Could you check a few things on this model? Use its own coordinates, in mm. Face numbers are marked on the shaded views. A direction names the side the tool comes from. Round coordinates to 2 decimals unless told otherwise and drop trailing zeros. Loops run counter-clockwise (first coordinate to the right, second up) from the corner with the lowest first, then second, coordinate; pieces in that order, holes last. Notation, with made-up numbers: (37, 46.25) -> (46, 46.25) arc R26 ccw to (46, 74.25) -> close; hole circle Ø3 at (83, -14). An arc over 180 degrees is marked (long way). One line per item, written item: value.
from build123d import *

# Parameters (mm, degrees)
P_IDAT_VYSUNUT_M2_DEPTH = 8


with BuildPart() as part:
    # Skica1 → Přidat vysunutím2 (new body)
    with BuildSketch(Plane(origin=(0, 0, 0), x_dir=(1, 0, 0), z_dir=(0, 1, 0))):
        with BuildLine():
            Line((0, -10), (0, 10))
            Line((0, 10), (5, 15))
            Line((5, 15), (36, 15))
            ThreePointArc((36, 15), (38.828427125, 16.171572875), (40, 19))
            Line((40, 19), (40, 25))
            Line((40, 25), (30, 25))
            Line((30, 25), (30, 20))
            Line((30, 20), (-13.506811582, 29.645227916))
            ThreePointArc((-13.506811582, 29.645227916), (-38.916330448, 23.640944379), (-49.997883531, 0))
            ThreePointArc((-49.997883531, 0), (-38.916330448, -23.640944379), (-13.506811582, -29.645227916))
            Line((-13.506811582, -29.645227916), (30, -20))
            Line((30, -20), (30, -25))
            Line((30, -25), (40, -25))
            Line((40, -25), (40, -19))
            ThreePointArc((40, -19), (38.828427125, -16.171572875), (36, -15))
            Line((36, -15), (5, -15))
            Line((5, -15), (0, -10))
        make_face()
    extrude(amount=P_IDAT_VYSUNUT_M2_DEPTH)


solid = part.part
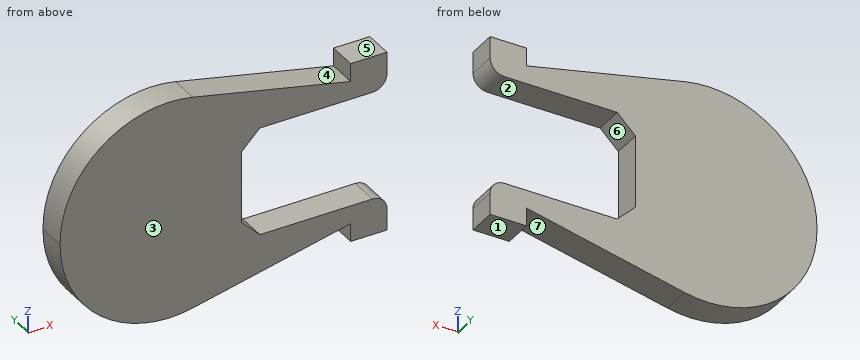
(1) If I drill on L1, parallel to Z at x = 31.5, y = 4.75; L2, parallel to X at y = 6, z = 0.5; L3, parallel to X at y = 4.75, z = 18, over which ranges is the centre line in solid material (lowest first)?
Recorded:
L1: -25 to -15, 15 to 25
L2: -50 to 0
L3: -44.26 to 39.87
(2) If we section it at A-A, the plane x = 34.5: Please give me the cut outline in (y, z).
Recorded:
outline: (0, -25) -> (8, -25) -> (8, -15) -> (0, -15) -> close; (0, 15) -> (8, 15) -> (8, 25) -> (0, 25) -> close
(3) If we section it at C-C, the plane y = 2: Please give me the cut outline in (x, z), then the cut area to 3 significant figures.
Recorded:
outline: (-50, 0) arc R30 ccw to (-13.51, -29.65) -> (30, -20) -> (30, -25) -> (40, -25) -> (40, -19) arc R4 ccw to (36, -15) -> (5, -15) -> (0, -10) -> (0, 10) -> (5, 15) -> (36, 15) arc R4 ccw to (40, 19) -> (40, 25) -> (30, 25) -> (30, 20) -> (-13.51, 29.65) arc R30 ccw to start
area: 3,300 mm²
(4) Thinking about a two-plate mould opening in Z: for the marked faces 5, 6 and 7, which applies, released by +Z, released by -Z, zero draft, split by the parting line, or undercut?
Recorded:
face 5: released by +Z
face 6: undercut
face 7: released by -Z
(5) If we section it at D-D, the plane z = -9: Please give me the cut outline in (x, y).
Recorded:
outline: (-48.73, 0) -> (0, 0) -> (0, 8) -> (-48.73, 8) -> close
(6) I'm going to push flat-ended pins straight in: pin 1 Ø1 at (y, z) = (1.5, -21) entering from -X; pin 2 Ø4 at (y, z) = (5, 21.5) entering from -X; pin 3 Ø1 at (y, z) = (2.5, 8.5) entering from -X. Where does each tip first touch, or does it pass through?
Recorded:
pin 1: x = -42.23
pin 2: x = -43.1
pin 3: x = -49.01
(7) If we section it at B-B, the plane z = 23: Please give me the cut outline in (x, y).
Recorded:
outline: (-39.68, 0) -> (16.47, 0) -> (16.47, 8) -> (-39.68, 8) -> close; (30, 0) -> (40, 0) -> (40, 8) -> (30, 8) -> close
(8) For the marked faces 1, 2, 3 and 4, which set-ups out of +Z, -Z, +X, -X, +Y, -Y let a thin tool reach every point of the face, with its end or its side?
Recorded:
face 1: -Z, +X, +Y, -Y
face 2: +X, +Y, -Y
face 3: +Z, -Z, +X, -X, -Y
face 4: +Z, +Y, -Y
